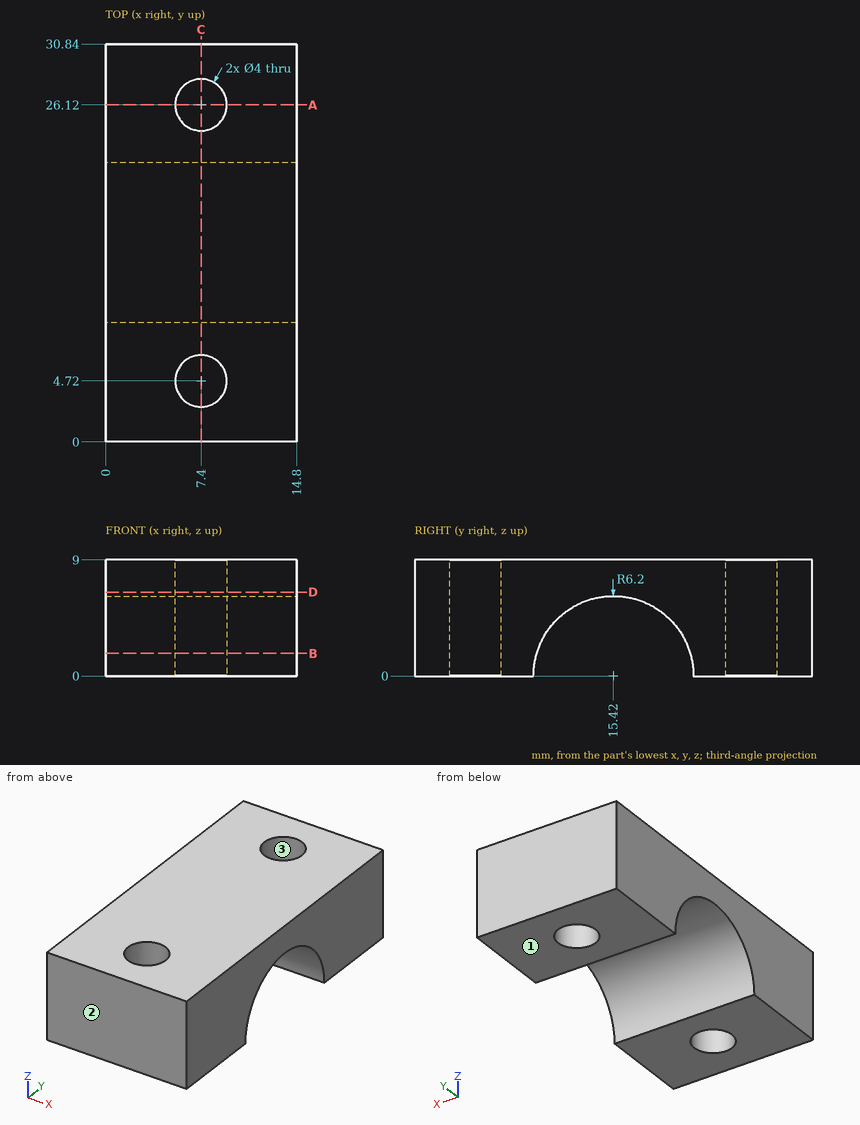
Study the drawing (mm; zero at the part's minimum x, y, z) and answer. Round coordinates to 2 decimals unless told otherwise and drop trailing zeros. Loops run counter-clockwise (first coordinate to the right, second up) from the corner with the lowest first, then second, coordinate; pieces in that order, holes last. Notation, with made-up numbers: (63, 57.5) - (87, 57.5) arc R17 ccw to (87, 76.5) - close; hole circle Ø3 at (17, 28). An arc over 180 degrees is marked (long way). Use one line per item in the form item = value. Start each with the question number.
1. The part is cut by section B-B on z = 1.75. Determine the outline of the cut face in (x, y), then the cut area to 3 significant figures.
2. Given pin 1 Ø2.5 at (x, y) = (7.4, 4.72) entering from -Z; pin 2 Ø1 at (x, y) = (7.5, 14.5) entering from -Z; pin 3 Ø2 at (x, y) = (12.5, 17.5) entering from -Z, each flat-ended and moving along its own axis, determine where each tip first touches the part or whether it passes through.
3. The part is cut by section D-D on z = 6.5. Determine the outline of the cut face in (x, y).
4. The part is cut by section C-C on x = 7.4. Determine the outline of the cut face in (y, z).
5. Consider line 1 (Y direction, x = 7.4, z = 6.5); line 2 (Y direction, x = 7.4, z = 4.25); line 3 (Y direction, x = 7.4, z = 5). Determine where each line is inside the solid, lowest interval first. Write a range as [from, to].
6. The part is cut by section A-A on y = 26.12. Determine the outline of the cut face in (x, z), then the cut area to 3 significant figures.
7. For a pull along Y with two mould halves and no side action, classify the marked faces 1, 2 and 3 as pulls with the +Y half, pulls with the -Y half, needs draft (parallel to the pull), parting line crosses it, or undercut.
Geometry check:
q1.outline = (0, 0) - (14.8, 0) - (14.8, 9.47) - (0, 9.47) - close; (0, 21.37) - (14.8, 21.37) - (14.8, 30.84) - (0, 30.84) - close; hole circle Ø4 at (7.4, 4.72); hole circle Ø4 at (7.4, 26.12)
q1.area = 255 mm^2
q2.pin_1 = through
q2.pin_2 = 6.04
q2.pin_3 = 5.38
q3.outline = (0, 0) - (14.8, 0) - (14.8, 30.84) - (0, 30.84) - close; hole circle Ø4 at (7.4, 4.72); hole circle Ø4 at (7.4, 26.12)
q4.outline = (0, 0) - (2.72, 0) - (2.72, 9) - (0, 9) - close; (6.72, 0) - (9.22, 0) arc R6.2 cw to (21.62, 0) - (24.12, 0) - (24.12, 9) - (6.72, 9) - close; (28.12, 0) - (30.84, 0) - (30.84, 9) - (28.12, 9) - close
q5.line_1 = [0, 2.72], [6.72, 24.12], [28.12, 30.84]
q5.line_2 = [0, 2.72], [6.72, 10.91], [19.93, 24.12], [28.12, 30.84]
q5.line_3 = [0, 2.72], [6.72, 11.75], [19.09, 24.12], [28.12, 30.84]
q6.outline = (0, 0) - (5.4, 0) - (5.4, 9) - (0, 9) - close; (9.4, 0) - (14.8, 0) - (14.8, 9) - (9.4, 9) - close
q6.area = 97.2 mm^2
q7.face_1 = needs draft
q7.face_2 = pulls with the -Y half
q7.face_3 = undercut
